Read the model definition and answer for the solid it produces. Units are mm, in the model's axes. A direction names the side the tool comes from. Coordinates: 2 decimals unless noted, no trailing zeros. Loops run counter-clockwise (first coordinate to the right, second up) from the corner with the lowest first, then second, coordinate; pieces in that order, holes last. Notation, with made-up numbers: (-32, -32.5) - (16, -32.5) arc R28 ccw to (16, 4.5) - close; hole circle Ø11 at (-36, 87). An arc over 180 degrees is marked (long way). Use CSV: the item, a comma, the result in double quotes.
```python
from build123d import *

# Parameters (mm, degrees)
SKETCH4_R      = 42.5
BASE_DEPTH     = 10
SKETCH5_R      = 5
SKETCH5_W      = 25
SKETCH5_H      = 40
TYRE_CUT_DEPTH = 10
SKETCH6_R      = 1.5
SKETCH6_R_2    = 2.5
NUTS_DEPTH     = 10


with BuildPart() as part:
    # Sketch4 → base (new body)
    with BuildSketch(Plane.XY):
        Circle(SKETCH4_R)
    extrude(amount=BASE_DEPTH)

    # Sketch5 → Tyre cut (cut)
    with BuildSketch(Plane.XY):
        Circle(SKETCH5_R)
        with Locations((0, 40)):
            Rectangle(SKETCH5_W, SKETCH5_H)
        Polygon((11.070508076, -20.825317547), (23.570508076, 0.825317547), (58.211524227, -19.174682453), (45.711524227, -40.825317547), align=None)
        Polygon((-23.570508076, 0.825317547), (-11.070508076, -20.825317547), (-45.711524227, -40.825317547), (-58.211524227, -19.174682453), align=None)
    extrude(amount=TYRE_CUT_DEPTH, mode=Mode.SUBTRACT)

    # Sketch6 → NUTs (cut)
    with BuildSketch(Plane.XY):
        with Locations((7.71570735, 16)):
            Circle(SKETCH6_R)
        with Locations((7.71570735, 4.825317547)):
            Circle(SKETCH6_R)
        with Locations(Location((34.527154016, 4.825317547, 0), (0, 0, 180))):
            Circle(SKETCH6_R)
        with Locations(Location((34.527154016, 16, 0), (0, 0, 180))):
            Circle(SKETCH6_R)
        with Locations((9.998552785, -14.681998573)):
            Circle(SKETCH6_R)
        with Locations((0.320993902, -9.094657347)):
            Circle(SKETCH6_R)
        with Locations(Location((-13.084729431, -32.314051272, 0), (0, 0, 180))):
            Circle(SKETCH6_R)
        with Locations(Location((-3.407170547, -37.901392498, 0), (0, 0, 180))):
            Circle(SKETCH6_R)
        with Locations((-17.714260136, -1.318001427)):
            Circle(SKETCH6_R)
        with Locations((-8.036701252, 4.2693398)):
            Circle(SKETCH6_R)
        with Locations(Location((-21.442424585, 27.488733725, 0), (0, 0, 180))):
            Circle(SKETCH6_R)
        with Locations(Location((-31.119983469, 21.901392498, 0), (0, 0, 180))):
            Circle(SKETCH6_R)
        with Locations((0, 12)):
            Circle(SKETCH6_R_2)
        with Locations((10.392304845, -6)):
            Circle(SKETCH6_R_2)
        with Locations((-10.392304845, -6)):
            Circle(SKETCH6_R_2)
        with Locations((31.472579283, 16)):
            Circle(SKETCH6_R)
        with Locations((31.472579283, 4.825317547)):
            Circle(SKETCH6_R)
        with Locations((4.672579283, 16)):
            Circle(SKETCH6_R)
        with Locations((4.672579283, 4.825317547)):
            Circle(SKETCH6_R)
        with Locations((11.520116819, -12.04657236)):
            Circle(SKETCH6_R)
        with Locations((1.842557936, -6.459231134)):
            Circle(SKETCH6_R)
        with Locations((-1.879883181, -35.256053181)):
            Circle(SKETCH6_R)
        with Locations((-11.557442064, -29.668711955)):
            Circle(SKETCH6_R)
        with Locations((-16.192696102, -3.95342764)):
            Circle(SKETCH6_R)
        with Locations((-6.515137219, 1.633913586)):
            Circle(SKETCH6_R)
        with Locations((-29.592696102, 19.256053181)):
            Circle(SKETCH6_R)
        with Locations((-19.915137219, 24.843394408)):
            Circle(SKETCH6_R)
    extrude(amount=NUTS_DEPTH, mode=Mode.SUBTRACT)


solid = part.part
```
Q1. For a pull along X with two mould halves and no side action, classify faces 1 (the face through (-36.6, 21.6, 4.9)), 2 (the face through (32.374, -4.258, 4.93)), 3 (the face through (9, 0, 10)), 4 (the face through (37.03, 20.86, 4.93)) as +X half, -X half, draft (parallel to the pull), parting line (faces both ways), or undercut.
Reported:
face 1,"-X half"
face 2,"undercut"
face 3,"draft"
face 4,"+X half"
Q2. The part is cut by section C-C on z = 8. Give the number of separate pieces and of enclosed holes in the cut face, and give its area (3 significant figures).
Reported:
separate pieces,"1"
enclosed holes,"28"
area,"3,730 mm²"
Q3. Given P1, Ø2.5, axis at x = 11.52, y = -12.05, coming from the -Z side; P2, Ø2, axis at y = 11, z = 3, coming from the -X side; P3, Ø6, axis at y = 14, z = 1.5, coming from the -X side; P4, Ø3, axis at x = -4.5, z = 5.5, coming from the +Y side, each flat-ended and moving along its own axis, determine where each tip first touches the part or whether it passes through.
Reported:
P1,"passes through"
P2,"stops at x = -41.31"
P3,"stops at x = -41.05"
P4,"stops at y = 20"
Q4. The part is cut by section A-A on x = 14. Determine the outline of the cut face in (y, z).
Reported:
outline,"(-40.13, 0) - (-22.52, 0) - (-22.52, 10) - (-40.13, 10) - close; (-15.75, 0) - (40.13, 0) - (40.13, 10) - (-15.75, 10) - close"
Q5. A tool of negligible diameter and unlimited length cuts with its end or side. For faces 5 (the face through (-19.874, -25.908, 4.93)), 6 (the face through (-17.408, -9.848, 4.93)), 7 (the face through (0, 20, 5)), from which of +Z, -Z, +X, -X, +Y, -Y can it reach the whole face along a straight path? Write none if from no direction.
Reported:
face 5,"+Z, -Z, -X"
face 6,"+Z, -Z"
face 7,"+Z, -Z, +Y"
Q6. Find the intervals of material crossed by probe 1 along Y at (x, z) = (-15, 8.75); probe 2 along Y at (x, z) = (35, 5.5); probe 3 along X at (y, z) = (1.5, 6.75), in increasing order. Write a range as [from, to].
Reported:
probe 1,"y = [-39.76, -23.09], [-14.02, -4.86], [-3.04, 39.76]"
probe 2,"y = [-5.77, 3.4], [6.25, 14.58], [17.42, 24.11]"
probe 3,"x = [-42.47, -8.01], [-5.02, -4.77], [4.77, 42.47]"
Q7. The part is cut by section B-B on y = 12. Determine the outline of the cut face in (x, z), and give its area (3 significant figures).
Reported:
outline,"(-40.77, 0) - (-2.5, 0) - (-2.5, 10) - (-40.77, 10) - close; (2.5, 0) - (40.77, 0) - (40.77, 10) - (2.5, 10) - close"
area,"765 mm²"
